For this review, take the finished solid that the model builds, in its own axes (mm). Coordinates: 2 decimals unless noted, no trailing zeros. Write each loop counter-clockwise with the first axis right and the second up, starting at its lowest first coordinate (ties: lowest second). Pieces come first, ordered by that corner, then holes.
1) We need section A-A on z = 22. Give the number of separate pieces and of enclosed holes in the cut face, then the cut area to 3 significant figures.
2) Insertion check: P1, Ø2, axis at x = -5, z = 87.5, coming from the -Y side. The pin has a flat end and moves straight along its axis. Give the tip position at first contact, or say it passes through.
3) To check wall thickness, follow line 1 along Z through (x, y) = (60, 2.95); line 2 along Z through (x, y) = (62, 1.15); line 3 along X through (y, z) = (3.15, 24.5). State the ranges of each line that lie inside material, in increasing order.
4) We need section B-B on x = -51.5. Write out the cut boundary in (y, z).
from build123d import *

# Parameters (mm, degrees)
SZKIC1_W                                          = 162.4
SZKIC1_H                                          = 180
DODANIE_WYCI_GNI_CIE1_DEPTH                       = 4
WYTNIJ_WYCI_GNI_CIE1_REACH                        = 123.282
SFAZOWANIE1_SIZE                                  = 4
POG_BIENIE_WALCOWE_POD_M3_RUB_Z_BEM_S_D           = 3.6
POG_BIENIE_WALCOWE_POD_M3_RUB_Z_BEM_S_DEPTH       = 6.7
POG_BIENIE_WALCOWE_POD_M3_RUB_Z_BEM_S_CBORE_D     = 7
POG_BIENIE_WALCOWE_POD_M3_RUB_Z_BEM_S_CBORE_DEPTH = 2.4
POG_BIENIE_WALCOWE_POD_M3_RUB_Z_BEM_S_TIP         = 1.081549114


with BuildPart() as part:
    # Szkic1 → Dodanie-wyciągnięcie1 (new body)
    with BuildSketch(Plane(origin=(0, 0, 0), x_dir=(1, 0, 0), z_dir=(0, 1, 0))):
        Rectangle(SZKIC1_W, SZKIC1_H)
    extrude(amount=DODANIE_WYCI_GNI_CIE1_DEPTH)

    # Szkic2 → Wytnij-wyciągnięcie1 (cut, up to next)
    with BuildSketch(Plane.XZ, mode=Mode.PRIVATE) as wytnij_wyci_gni_cie1_sk1:
        with BuildLine():
            Line((-44, -47.828427125), (-44, -67.171572875))
            add(Edge.make_bspline(
                [(-46, -70), (-44, -70), (-44, -67.171572875)],
                knots=[3.141592654, 3.141592654, 3.141592654, 4.71238898, 4.71238898, 4.71238898], degree=2, weights=[1, 0.707106781, 1]))
            Line((-46, -70), (-67, -70))
            add(Edge.make_bspline(
                [(-69, -67.171572875), (-69, -70), (-67, -70)],
                knots=[1.570796327, 1.570796327, 1.570796327, 3.141592654, 3.141592654, 3.141592654], degree=2, weights=[1, 0.707106781, 1]))
            Line((-69, -67.171572875), (-69, -47.828427125))
            add(Edge.make_bspline(
                [(-67, -45), (-69, -45), (-69, -47.828427125)],
                knots=[0, 0, 0, 1.570796327, 1.570796327, 1.570796327], degree=2, weights=[1, 0.707106781, 1]))
            Line((-67, -45), (-46, -45))
            add(Edge.make_bspline(
                [(-44, -47.828427125), (-44, -45), (-46, -45)],
                knots=[4.71238898, 4.71238898, 4.71238898, 6.283185307, 6.283185307, 6.283185307], degree=2, weights=[1, 0.707106781, 1]))
        make_face()
    wytnij_wyci_gni_cie1_tool1 = extrude(wytnij_wyci_gni_cie1_sk1.sketch, amount=-WYTNIJ_WYCI_GNI_CIE1_REACH, mode=Mode.PRIVATE) & part.part
    # Szkic2 → Wytnij-wyciągnięcie1 (cut, up to next)
    with BuildSketch(Plane.XZ, mode=Mode.PRIVATE) as wytnij_wyci_gni_cie1_sk2:
        with BuildLine():
            Line((10, -47.828427125), (10, -67.171572875))
            add(Edge.make_bspline(
                [(8, -70), (10, -70), (10, -67.171572875)],
                knots=[3.141592654, 3.141592654, 3.141592654, 4.71238898, 4.71238898, 4.71238898], degree=2, weights=[1, 0.707106781, 1]))
            Line((8, -70), (-13, -70))
            add(Edge.make_bspline(
                [(-15, -67.171572875), (-15, -70), (-13, -70)],
                knots=[1.570796327, 1.570796327, 1.570796327, 3.141592654, 3.141592654, 3.141592654], degree=2, weights=[1, 0.707106781, 1]))
            Line((-15, -67.171572875), (-15, -47.828427125))
            add(Edge.make_bspline(
                [(-13, -45), (-15, -45), (-15, -47.828427125)],
                knots=[0, 0, 0, 1.570796327, 1.570796327, 1.570796327], degree=2, weights=[1, 0.707106781, 1]))
            Line((-13, -45), (8, -45))
            add(Edge.make_bspline(
                [(10, -47.828427125), (10, -45), (8, -45)],
                knots=[4.71238898, 4.71238898, 4.71238898, 6.283185307, 6.283185307, 6.283185307], degree=2, weights=[1, 0.707106781, 1]))
        make_face()
    wytnij_wyci_gni_cie1_tool2 = extrude(wytnij_wyci_gni_cie1_sk2.sketch, amount=-WYTNIJ_WYCI_GNI_CIE1_REACH, mode=Mode.PRIVATE) & part.part
    # Szkic2 → Wytnij-wyciągnięcie1 (cut, up to next)
    with BuildSketch(Plane.XZ, mode=Mode.PRIVATE) as wytnij_wyci_gni_cie1_sk3:
        Polygon((-9.2, -33), (5.3, -33), (5.3, 1), (15.3, 1), (15.3, -80), (20.3, -80), (20.3, 63), (15.3, 63), (15.3, 38), (5.3, 38), (5.3, 68), (-9.2, 68), align=None)
    wytnij_wyci_gni_cie1_tool3 = extrude(wytnij_wyci_gni_cie1_sk3.sketch, amount=-WYTNIJ_WYCI_GNI_CIE1_REACH, mode=Mode.PRIVATE) & part.part
    # Szkic2 → Wytnij-wyciągnięcie1 (cut, up to next)
    with BuildSketch(Plane.XZ, mode=Mode.PRIVATE) as wytnij_wyci_gni_cie1_sk4:
        Polygon((-63.2, -33), (-48.7, -33), (-48.7, 1), (-38.7, 1), (-38.7, -80), (-33.7, -80), (-33.7, 63), (-38.7, 63), (-38.7, 38), (-48.7, 38), (-48.7, 68), (-63.2, 68), align=None)
    wytnij_wyci_gni_cie1_tool4 = extrude(wytnij_wyci_gni_cie1_sk4.sketch, amount=-WYTNIJ_WYCI_GNI_CIE1_REACH, mode=Mode.PRIVATE) & part.part
    # Szkic2 → Wytnij-wyciągnięcie1 (cut, up to next)
    with BuildSketch(Plane.XZ, mode=Mode.PRIVATE) as wytnij_wyci_gni_cie1_sk5:
        with BuildLine():
            Line((64, -47.828427125), (64, -67.171572875))
            add(Edge.make_bspline(
                [(62, -70), (64, -70), (64, -67.171572875)],
                knots=[3.141592654, 3.141592654, 3.141592654, 4.71238898, 4.71238898, 4.71238898], degree=2, weights=[1, 0.707106781, 1]))
            Line((62, -70), (41, -70))
            add(Edge.make_bspline(
                [(39, -67.171572875), (39, -70), (41, -70)],
                knots=[1.570796327, 1.570796327, 1.570796327, 3.141592654, 3.141592654, 3.141592654], degree=2, weights=[1, 0.707106781, 1]))
            Line((39, -67.171572875), (39, -47.828427125))
            add(Edge.make_bspline(
                [(41, -45), (39, -45), (39, -47.828427125)],
                knots=[0, 0, 0, 1.570796327, 1.570796327, 1.570796327], degree=2, weights=[1, 0.707106781, 1]))
            Line((41, -45), (62, -45))
            add(Edge.make_bspline(
                [(64, -47.828427125), (64, -45), (62, -45)],
                knots=[4.71238898, 4.71238898, 4.71238898, 6.283185307, 6.283185307, 6.283185307], degree=2, weights=[1, 0.707106781, 1]))
        make_face()
    wytnij_wyci_gni_cie1_tool5 = extrude(wytnij_wyci_gni_cie1_sk5.sketch, amount=-WYTNIJ_WYCI_GNI_CIE1_REACH, mode=Mode.PRIVATE) & part.part
    # Szkic2 → Wytnij-wyciągnięcie1 (cut, up to next)
    with BuildSketch(Plane.XZ, mode=Mode.PRIVATE) as wytnij_wyci_gni_cie1_sk6:
        Polygon((44.8, -33), (59.3, -33), (59.3, 1), (69.3, 1), (69.3, -80), (74.3, -80), (74.3, 63), (69.3, 63), (69.3, 38), (59.3, 38), (59.3, 68), (44.8, 68), align=None)
    wytnij_wyci_gni_cie1_tool6 = extrude(wytnij_wyci_gni_cie1_sk6.sketch, amount=-WYTNIJ_WYCI_GNI_CIE1_REACH, mode=Mode.PRIVATE) & part.part
    add(wytnij_wyci_gni_cie1_tool1.solids().sort_by_distance((-56.5, 0, -57.5))[0], mode=Mode.SUBTRACT)
    add(wytnij_wyci_gni_cie1_tool2.solids().sort_by_distance((-2.5, 0, -57.5))[0], mode=Mode.SUBTRACT)
    add(wytnij_wyci_gni_cie1_tool3.solids().sort_by_distance((5.366631, 0, 10.498627))[0], mode=Mode.SUBTRACT)
    add(wytnij_wyci_gni_cie1_tool4.solids().sort_by_distance((-48.633369, 0, 10.498627))[0], mode=Mode.SUBTRACT)
    add(wytnij_wyci_gni_cie1_tool5.solids().sort_by_distance((51.5, 0, -57.5))[0], mode=Mode.SUBTRACT)
    add(wytnij_wyci_gni_cie1_tool6.solids().sort_by_distance((59.366631, 0, 10.498627))[0], mode=Mode.SUBTRACT)

    # Sfazowanie1
    sfazowanie1_edges = [part.edges().sort_by_distance(p)[0] for p in [
        (69.3, 4, -39.5),
        (74.3, 4, -8.5),
        (69.3, 4, 50.5),
        (59.3, 4, 53),
        (59.3, 4, -16),
        (44.8, 4, 17.5),
        (15.3, 4, -39.5),
        (15.3, 4, 50.5),
        (20.3, 4, -8.5),
        (5.3, 4, 53),
        (5.3, 4, -16),
        (-9.2, 4, 17.5),
        (-33.7, 4, -8.5),
        (-38.7, 4, -39.5),
        (-38.7, 4, 50.5),
        (-48.7, 4, 53),
        (-48.7, 4, -16),
        (-63.2, 4, 17.5),
    ]]
    chamfer(sfazowanie1_edges, length=SFAZOWANIE1_SIZE - 0.0001)  # a hair under: the kernel refuses the full size

    # Pogłębienie walcowe pod M3 Śrubę z łbem stożkowym ściętym1
    with Locations(Plane.XZ):
        with Locations((77.6, 86.4), (77.6, -86.4), (50.16, -86.4), (22.72, -86.4), (-4.72, -86.4), (-32.16, -86.4), (-59.6, -86.4), (-59.6, 86.4), (-32.16, 86.4), (-4.72, 86.4), (22.72, 86.4), (50.16, 86.4)):
            CounterBoreHole(POG_BIENIE_WALCOWE_POD_M3_RUB_Z_BEM_S_D / 2, POG_BIENIE_WALCOWE_POD_M3_RUB_Z_BEM_S_CBORE_D / 2, POG_BIENIE_WALCOWE_POD_M3_RUB_Z_BEM_S_CBORE_DEPTH, depth=POG_BIENIE_WALCOWE_POD_M3_RUB_Z_BEM_S_DEPTH)
            with Locations((0, 0, -(POG_BIENIE_WALCOWE_POD_M3_RUB_Z_BEM_S_DEPTH + POG_BIENIE_WALCOWE_POD_M3_RUB_Z_BEM_S_TIP / 2))):  # 118° drill point
                Cone(0, POG_BIENIE_WALCOWE_POD_M3_RUB_Z_BEM_S_D / 2, POG_BIENIE_WALCOWE_POD_M3_RUB_Z_BEM_S_TIP, mode=Mode.SUBTRACT)


solid = part.part
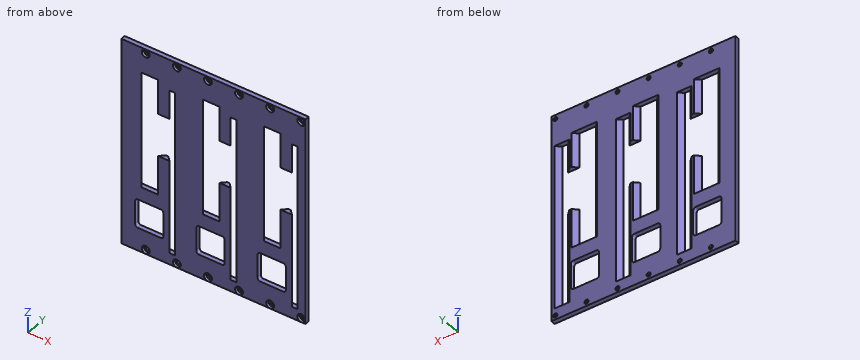
Result:
1. separate pieces: 4
1. enclosed holes: 0
1. area: 248 mm2
2. P1: stops at y = 2.4
3. line 1: z = -90 to -70, -45 to -33, 68 to 90
3. line 2: z = -90 to -70, -45 to 1, 38 to 90
3. line 3: x = -81.2 to -66.35, -30.55 to -12.35, 23.45 to 41.65, 77.45 to 81.2
4. outline: (0, -90) - (4, -90) - (4, -70) - (0, -70) - close; (0, -45) - (4, -45) - (4, -33) - (0, -33) - close; (0, 68) - (4, 68) - (4, 90) - (0, 90) - close
